```python
from build123d import *

# Parameters (mm, degrees)
SKETCH1_R           = 1.6
SKETCH1_R_2         = 3
BOSS_EXTRUDE1_DEPTH = 10
BOSS_EXTRUDE2_DEPTH = 5
SKETCH3_R           = 1.6
CUT_EXTRUDE2_DEPTH  = 24
FILLET1_R           = 10
SKETCH4_W           = 29.614558854
SKETCH4_H           = 6.006759352
BOSS_EXTRUDE3_DEPTH = 15
FILLET2_R           = 10
SKETCH5_R           = 1.6
CUT_EXTRUDE3_DEPTH  = 15


with BuildPart() as part:
    # Sketch1 → Boss-Extrude1 (new body)
    with BuildSketch(Plane(origin=(0, 0, 0), x_dir=(1, 0, 0), z_dir=(0, 1, 0))):
        with BuildLine():
            Line((13.581493994, 58.752113328), (-10.918506006, 58.752113328))
            ThreePointArc((-10.918506006, 58.752113328), (-17.989573818, 61.681045517), (-20.918506006, 68.752113328))
            Line((-20.918506006, 68.752113328), (-20.918506006, 72.587513875))
            ThreePointArc((-20.918506006, 72.587513875), (-21.797185662, 74.708834218), (-23.918506006, 75.587513875))
            Line((-23.918506006, 75.587513875), (-44.093226465, 75.587513875))
            ThreePointArc((-44.093226465, 75.587513875), (-46.214546809, 74.708834218), (-47.093226465, 72.587513875))
            Line((-47.093226465, 72.587513875), (-47.093226465, 44.912793415))
            ThreePointArc((-47.093226465, 44.912793415), (-46.566018672, 43.640001209), (-45.293226465, 43.112793415))
            Line((-45.293226465, 43.112793415), (-45.277758982, 43.112793415))
            ThreePointArc((-45.277758982, 43.112793415), (-38.20669117, 40.183861227), (-35.277758982, 33.112793415))
            Line((-35.277758982, 33.112793415), (-35.277758982, -34.387206585))
            ThreePointArc((-35.277758982, -34.387206585), (-38.20669117, -41.458274396), (-45.277758982, -44.387206585))
            Line((-45.277758982, -44.387206585), (-45.293226465, -44.387206585))
            ThreePointArc((-45.293226465, -44.387206585), (-46.566018672, -44.914414378), (-47.093226465, -46.187206585))
            Line((-47.093226465, -46.187206585), (-47.093226465, -73.861927044))
            ThreePointArc((-47.093226465, -73.861927044), (-46.214546809, -75.983247388), (-44.093226465, -76.861927044))
            Line((-44.093226465, -76.861927044), (46.756214453, -76.861927044))
            ThreePointArc((46.756214453, -76.861927044), (48.877534797, -75.983247388), (49.756214453, -73.861927044))
            Line((49.756214453, -73.861927044), (49.756214453, -46.187206585))
            ThreePointArc((49.756214453, -46.187206585), (49.22900666, -44.914414378), (47.956214453, -44.387206585))
            Line((47.956214453, -44.387206585), (47.94130771, -44.387206585))
            ThreePointArc((47.94130771, -44.387206585), (40.870239898, -41.458274396), (37.94130771, -34.387206585))
            Line((37.94130771, -34.387206585), (37.94130771, 33.112793415))
            ThreePointArc((37.94130771, 33.112793415), (40.870239898, 40.183861227), (47.94130771, 43.112793415))
            Line((47.94130771, 43.112793415), (47.956214453, 43.112793415))
            ThreePointArc((47.956214453, 43.112793415), (49.22900666, 43.640001209), (49.756214453, 44.912793415))
            Line((49.756214453, 44.912793415), (49.756214453, 72.587513875))
            ThreePointArc((49.756214453, 72.587513875), (48.877534797, 74.708834218), (46.756214453, 75.587513875))
            Line((46.756214453, 75.587513875), (26.581493994, 75.587513875))
            ThreePointArc((26.581493994, 75.587513875), (24.46017365, 74.708834218), (23.581493994, 72.587513875))
            Line((23.581493994, 72.587513875), (23.581493994, 68.752113328))
            ThreePointArc((23.581493994, 68.752113328), (20.652561806, 61.681045517), (13.581493994, 58.752113328))
        make_face()
        with Locations(Location((-42.755866236, -47.524566814, 0), (0, 0, 90))):
            Circle(SKETCH1_R, mode=Mode.SUBTRACT)
        with Locations(Location((-25.255866236, -47.524566814, 0), (0, 0, 90))):
            Circle(SKETCH1_R, mode=Mode.SUBTRACT)
        with Locations(Location((-25.255866236, -72.524566814, 0), (0, 0, 90))):
            Circle(SKETCH1_R, mode=Mode.SUBTRACT)
        with Locations(Location((-42.755866236, -72.524566814, 0), (0, 0, 90))):
            Circle(SKETCH1_R, mode=Mode.SUBTRACT)
        Polygon((-15.746148386, 7.031408071), (18.409136374, 7.031408071), (22.481493994, 3.156595611), (22.481493994, -31.29377947), (18.506681534, -35.268591929), (7.482919934, -35.268591929), (7.482919934, -43.496504735), (-4.819931946, -43.496504735), (-4.819931946, -35.268591929), (-15.843693546, -35.268591929), (-19.818506006, -31.29377947), (-19.818506006, 3.156595611), align=None, mode=Mode.SUBTRACT)
        with Locations(Location((45.418854224, -72.524566814, 0), (0, 0, 270))):
            Circle(SKETCH1_R, mode=Mode.SUBTRACT)
        with Locations(Location((27.918854224, -72.524566814, 0), (0, 0, 270))):
            Circle(SKETCH1_R, mode=Mode.SUBTRACT)
        with Locations(Location((27.918854224, -47.524566814, 0), (0, 0, 270))):
            Circle(SKETCH1_R, mode=Mode.SUBTRACT)
        with Locations(Location((45.418854224, -47.524566814, 0), (0, 0, 270))):
            Circle(SKETCH1_R, mode=Mode.SUBTRACT)
        with Locations(Location((1.331493994, 29.261782359, 0), (0, 0, 270))):
            Circle(SKETCH1_R_2, mode=Mode.SUBTRACT)
        with Locations(Location((-42.755866236, 71.250153645, 0), (0, 0, 270))):
            Circle(SKETCH1_R, mode=Mode.SUBTRACT)
        with Locations(Location((-42.755866236, 46.250153645, 0), (0, 0, 270))):
            Circle(SKETCH1_R, mode=Mode.SUBTRACT)
        with Locations(Location((-25.255866236, 46.250153645, 0), (0, 0, 270))):
            Circle(SKETCH1_R, mode=Mode.SUBTRACT)
        with Locations(Location((-25.255866236, 71.250153645, 0), (0, 0, 270))):
            Circle(SKETCH1_R, mode=Mode.SUBTRACT)
        with Locations(Location((27.918854224, 46.250153645, 0), (0, 0, 90))):
            Circle(SKETCH1_R, mode=Mode.SUBTRACT)
        with Locations(Location((27.918854224, 71.250153645, 0), (0, 0, 90))):
            Circle(SKETCH1_R, mode=Mode.SUBTRACT)
        with Locations(Location((45.418854224, 71.250153645, 0), (0, 0, 90))):
            Circle(SKETCH1_R, mode=Mode.SUBTRACT)
        with Locations(Location((45.418854224, 46.250153645, 0), (0, 0, 90))):
            Circle(SKETCH1_R, mode=Mode.SUBTRACT)
    extrude(amount=BOSS_EXTRUDE1_DEPTH)

    # Sketch1<3> → Boss-Extrude2 (add)
    with BuildSketch(Plane(origin=(0, 0, 0), x_dir=(1, 0, 0), z_dir=(0, 1, 0))):
        Polygon((18.409136374, 7.031408071), (-15.746148386, 7.031408071), (-19.818506006, 3.156595611), (-19.818506006, -31.29377947), (-15.843693546, -35.268591929), (-4.819931946, -35.268591929), (-4.819931946, -43.496504735), (7.482919934, -43.496504735), (7.482919934, -35.268591929), (18.506681534, -35.268591929), (22.481493994, -31.29377947), (22.481493994, 3.156595611), align=None)
    extrude(amount=BOSS_EXTRUDE2_DEPTH)

    # Sketch3 → Cut-Extrude2 (cut)
    with BuildSketch(Plane(origin=(0, 10, 0), x_dir=(1, 0, 0), z_dir=(0, 1, 0))):
        with Locations(Location((-24.902167588, -40.352253511, 0), (0, 0, 270))):
            Circle(SKETCH3_R)
        with Locations(Location((27.565155576, -40.352253511, 0), (0, 0, 90))):
            Circle(SKETCH3_R)
        with Locations(Location((27.565155576, 12.115069653, 0), (0, 0, 270))):
            Circle(SKETCH3_R)
        with Locations(Location((-24.902167588, 12.115069653, 0), (0, 0, 90))):
            Circle(SKETCH3_R)
    extrude(amount=-CUT_EXTRUDE2_DEPTH, mode=Mode.SUBTRACT)

    # Fillet1
    fillet1_edges = [part.edges().sort_by_distance(p)[0] for p in [
        (1.331493994, 10, -32.261782359),
    ]]
    fillet(fillet1_edges, radius=FILLET1_R - 0.0001)  # a hair under: the kernel refuses the full size

    # Sketch4 → Boss-Extrude3 (add)
    with BuildSketch(Plane(origin=(0, 10, 0), x_dir=(1, 0, 0), z_dir=(0, 1, 0))):
        with Locations((1.331493994, -73.858547368)):
            Rectangle(SKETCH4_W, SKETCH4_H)
    extrude(amount=BOSS_EXTRUDE3_DEPTH)

    # Fillet2
    fillet2_edges = [part.edges().sort_by_distance(p)[0] for p in [
        (16.138773421, 25, 73.858547368),
        (-13.475785433, 25, 73.858547368),
    ]]
    fillet(fillet2_edges, radius=FILLET2_R)

    # Sketch5 → Cut-Extrude3 (cut)
    with BuildSketch(Plane.XY.offset(76.861927044)):
        with Locations((1.331493994, 19.855091715)):
            Circle(SKETCH5_R)
    extrude(amount=-CUT_EXTRUDE3_DEPTH, mode=Mode.SUBTRACT)


solid = part.part
```
The model under review builds one solid part; all positions refer to its coordinate system, in mm. A direction names the side the tool comes from. Give positions to 0.01 mm unless a question says otherwise; leave off trailing zeros. Loops run counter-clockwise (first coordinate to the right, second up) from the corner with the lowest first, then second, coordinate; pieces in that order, holes last. Notation, with made-up numbers: (78.25, 22) - (132.25, 22) arc R16 ccw to (132.25, 35) - close; hole circle Ø10 at (42.5, 19). An arc over 180 degrees is marked (long way). Answer as a JSON object with one key per item and string values.
Q1. Add section D-D on z = -51. State the section outline as (x, y) points, plus the area to 3 significant figures.
Worked out:
{"outline": "(-47.09, 0) - (49.76, 0) - (49.76, 10) - (-47.09, 10) - close", "area": "968 mm^2"}
Q2. Add section A-A on x = -37. State the section outline as (y, z) points.
Worked out:
{"outline": "(0, -75.59) - (10, -75.59) - (10, -38.72) - (0, -38.72) - close; (0, 40) - (10, 40) - (10, 76.86) - (0, 76.86) - close"}
Q3. Add section C-C on x = 31.5. State the section outline as (y, z) points, plus the area to 3 significant figures.
Worked out:
{"outline": "(0, -75.59) - (10, -75.59) - (10, 76.86) - (0, 76.86) - close", "area": "1,520 mm^2"}
Q4. For faces 4 (the flat face through (-13.476, 12, 74)), 5 (the cylindrical face through (-21.774, 4.93, -74.685)), 6 (the cylindrical face through (29.338, 4.93, -71.988)), 7 (the flat face through (20.42, 7.46, -5.12)), 8 (the flat face through (1, 17, 70.855)), list the 3-axis set-ups (+Z, -Z, +X, -X, +Y, -Y) from which the entire face can be reached by the end or side of a thin tool; tool diameter is ignored.
Worked out:
{"face 4": "+Z, -Z, -X, +Y", "face 5": "-Z, +Y, -Y", "face 6": "+Y, -Y", "face 7": "+Y", "face 8": "-Z, +X, -X, +Y"}
Q5. Insertion check: pin 1 (8 mm diameter, centred on y = 11.5, z = 17.5, fed in from +X); pin 2 (4 mm diameter, centred on x = 27.92, z = 47.52, fed in from +Y); pin 3 (2.5 mm diameter, centred on x = -10, y = 7, fed in from -Z); pin 4 (12 mm diameter, centred on x = 38.5, y = 20, fed in from +Z). Each pin has a flat end and moves straight along its axis. Give the tip position at first contact, or say it passes through.
Worked out:
{"pin 1": "stops at x = 37.94", "pin 2": "stops at y = 10", "pin 3": "stops at z = -58.76", "pin 4": "passes through"}
Q6. Mouldability with a two-part tool opening along Z and no side actions: class faces 1 (the flat face through (1, 0, 0)), 2 (the flat face through (37, 5, -75.588)), 3 (the flat face through (20.522, 7.465, 33.253)) as +Z half, -Z half, draft (parallel to the pull), parting line (faces both ways), or undercut.
Worked out:
{"face 1": "draft", "face 2": "-Z half", "face 3": "undercut"}
Q7. To check wall thickness, follow line 1 along Z through (x, y) = (-8, 7.5); line 2 along Y through (x, z) = (-14, 14); line 3 along Y through (x, z) = (-30, 24). State the ranges of each line that lie inside material, in increasing order.
Worked out:
{"line 1": "z = -58.75 to -7.03, 35.27 to 76.86", "line 2": "y = 0 to 5", "line 3": "y = 0 to 10"}
Q8. Add section B-B on z = 18. State the section outline as (x, y) points.
Worked out:
{"outline": "(-35.28, 0) - (37.94, 0) - (37.94, 10) - (22.48, 10) - (22.48, 5) - (-19.82, 5) - (-19.82, 10) - (-35.28, 10) - close"}
